CAD build for the part. Positions are in the model's coordinates, mm. Face numbers are marked on the shaded views. A direction names the side the tool comes from. Give positions to 0.01 mm unless a question says otherwise; leave off trailing zeros. Write each loop counter-clockwise with the first axis right and the second up, starting at its lowest first coordinate (ties: lowest second). Pieces come first, ordered by that corner, then holes. Notation, with made-up numbers: (-37, -1) -> (6, -1) arc R18 cw to (6, 26) -> close; hole circle Ø5 at (46, -11). An arc over 180 degrees is marked (long way). Answer as a JSON object with one key per item and string values.
```python
from build123d import *

# Parameters (mm, degrees)
F0_W     = 25
F0_H     = 38
F1_DEPTH = 5
F3_DEPTH = 5
F5_DEPTH = 15.5
F7_DEPTH = 25
F8_R     = 1.9
F9_DEPTH = 1


# Not quite as in the source:
# - a feature names something its author has since deleted; it is built from what else it names


with BuildPart() as f1:
    # F0 (on Top) → F1 (new body)
    with BuildSketch(Plane.XY):
        with Locations((-5.6626851261, 7.8445598302)):
            Rectangle(F0_W, F0_H)
    extrude(amount=F1_DEPTH)

    # F2 (on face) → F3 (cut)
    with BuildSketch(Plane.XY.offset(5)):
        with BuildLine():
            Line((-13.6626851261, 15.8445598302), (-12.5876851261, 15.8445598302))
            ThreePointArc((-12.5876851261, 15.8445598302), (-14.4228249158, 16.60469962), (-13.6626851261, 14.7695598302))
            Line((-13.6626851261, 14.7695598302), (-13.6626851261, 15.8445598302))
        make_face()
        with BuildLine():
            ThreePointArc((-13.6626851261, 14.7695598302), (-12.9025453363, 15.0844200404), (-12.5876851261, 15.8445598302))
            Line((-12.5876851261, 15.8445598302), (-13.6626851261, 15.8445598302))
            Line((-13.6626851261, 15.8445598302), (-13.6626851261, 14.7695598302))
        make_face()
        with BuildLine():
            Line((2.3373148739, 15.8445598302), (1.2623148739, 15.8445598302))
            ThreePointArc((1.2623148739, 15.8445598302), (1.5771750842, 15.0844200404), (2.3373148739, 14.7695598302))
            Line((2.3373148739, 14.7695598302), (2.3373148739, 15.8445598302))
        make_face()
        with BuildLine():
            ThreePointArc((3.4123148739, 15.8445598302), (2.3373148739, 16.9195598302), (1.2623148739, 15.8445598302))
            Line((1.2623148739, 15.8445598302), (2.3373148739, 15.8445598302))
            Line((2.3373148739, 15.8445598302), (2.3373148739, 14.7695598302))
            ThreePointArc((2.3373148739, 14.7695598302), (3.0974546637, 15.0844200404), (3.4123148739, 15.8445598302))
        make_face()
        with BuildLine():
            Line((-13.6626851261, -0.1554401698), (-13.6626851261, 0.9195598302))
            ThreePointArc((-13.6626851261, 0.9195598302), (-14.4228249158, -0.9155799596), (-12.5876851261, -0.1554401698))
            Line((-12.5876851261, -0.1554401698), (-13.6626851261, -0.1554401698))
        make_face()
        with BuildLine():
            ThreePointArc((-12.5876851261, -0.1554401698), (-12.9025453363, 0.60469962), (-13.6626851261, 0.9195598302))
            Line((-13.6626851261, 0.9195598302), (-13.6626851261, -0.1554401698))
            Line((-13.6626851261, -0.1554401698), (-12.5876851261, -0.1554401698))
        make_face()
        with BuildLine():
            Line((2.3373148739, -0.1554401698), (2.3373148739, 0.9195598302))
            ThreePointArc((2.3373148739, 0.9195598302), (1.5771750842, 0.60469962), (1.2623148739, -0.1554401698))
            Line((1.2623148739, -0.1554401698), (2.3373148739, -0.1554401698))
        make_face()
        with BuildLine():
            ThreePointArc((3.4123148739, -0.1554401698), (3.0974546637, 0.60469962), (2.3373148739, 0.9195598302))
            Line((2.3373148739, 0.9195598302), (2.3373148739, -0.1554401698))
            Line((2.3373148739, -0.1554401698), (1.2623148739, -0.1554401698))
            ThreePointArc((1.2623148739, -0.1554401698), (2.3373148739, -1.2304401698), (3.4123148739, -0.1554401698))
        make_face()
    extrude(amount=-F3_DEPTH, mode=Mode.SUBTRACT)

    # F4 (on face) → F5 (join)
    with BuildSketch(Plane.XY.offset(5)):
        Polygon((-15.2126851261, 13.8445598302), (-15.2126851261, 1.8445598302), (-14.2126851261, 1.8445598302), (-13.2126851261, 1.8445598302), (-13.2126851261, 13.8445598302), (-14.2126851261, 13.8445598302), align=None)
        Polygon((4.0873148739, 13.8445598302), (3.0873148739, 13.8445598302), (2.0873148739, 13.8445598302), (2.0873148739, 1.8445598302), (4.0873148739, 1.8445598302), align=None)
    extrude(amount=F5_DEPTH)

    # F6 (on face) → F7 (cut)
    with BuildSketch(Plane.YZ.offset(4.0873148739)):
        with BuildLine():
            Line((7.8445598302, 11.45), (7.8445598302, 14.55))
            ThreePointArc((7.8445598302, 14.55), (6.2945598302, 13), (7.8445598302, 11.45))
        make_face()
        with BuildLine():
            ThreePointArc((7.8445598302, 11.45), (8.9405753411, 11.9039844892), (9.3945598302, 13))
            ThreePointArc((9.3945598302, 13), (8.9405753411, 14.0960155108), (7.8445598302, 14.55))
            Line((7.8445598302, 14.55), (7.8445598302, 11.45))
        make_face()
    extrude(amount=-F7_DEPTH, mode=Mode.SUBTRACT)

    # F8 (on face) → F9 (cut)
    with BuildSketch(Plane.XY.offset(5)):
        with Locations((-13.6626851261, 15.8445598302)):
            Circle(F8_R)
        with Locations((2.3373148739, 15.8445598302)):
            Circle(F8_R)
        with Locations((2.3373148739, -0.1554401698)):
            Circle(F8_R)
        with Locations((-13.6626851261, -0.1554401698)):
            Circle(F8_R)
    extrude(amount=-F9_DEPTH, mode=Mode.SUBTRACT)


solid = f1.part
```
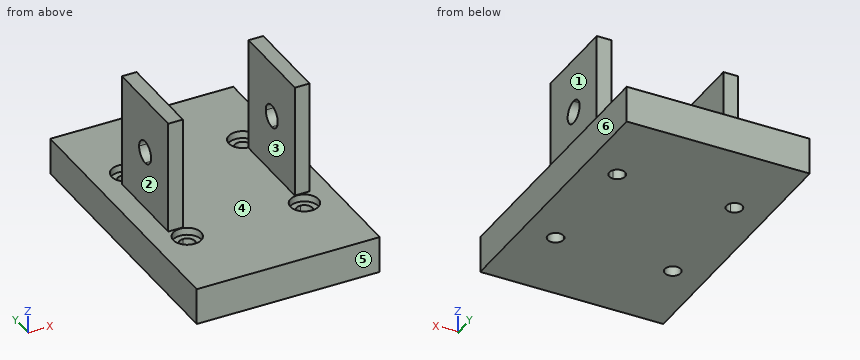
1) Slice it at B-B (z = 2.75). List the corners of the cut face in (x, y) (3 decimals).
Model answer:
{"outline": "(-18.163, -11.155) -> (6.837, -11.155) -> (6.837, 26.845) -> (-18.163, 26.845) -> close; hole circle Ø2.15 at (-13.663, -0.155); hole circle Ø2.15 at (-13.663, 15.845); hole circle Ø2.15 at (2.337, -0.155); hole circle Ø2.15 at (2.337, 15.845)"}
2) Wall check: probe 1 along X at (y, z) = (4, 13.75); probe 2 along Z at (x, y) = (2.5, 24.5); probe 3 along Y at (x, z) = (-13.5, 5.5). Give the ranges that are in metal, low to high.
Model answer:
{"probe 1": "x = -15.21 to -13.21, 2.09 to 4.09", "probe 2": "z = 0 to 5", "probe 3": "y = 1.84 to 13.84"}
3) Slice it at C-C (y = 5.5). List the corners of the cut face in (x, z).
Model answer:
{"outline": "(-18.16, 0) -> (6.84, 0) -> (6.84, 5) -> (4.09, 5) -> (4.09, 20.5) -> (2.09, 20.5) -> (2.09, 5) -> (-13.21, 5) -> (-13.21, 20.5) -> (-15.21, 20.5) -> (-15.21, 5) -> (-18.16, 5) -> close"}
4) Slice it at A-A (z = 7.25). List the corners of the cut face in (x, y).
Model answer:
{"outline": "(-15.21, 1.84) -> (-13.21, 1.84) -> (-13.21, 13.84) -> (-15.21, 13.84) -> close; (2.09, 1.84) -> (4.09, 1.84) -> (4.09, 13.84) -> (2.09, 13.84) -> close"}
5) 3-axis set-ups, long thin cutter, end or side, ignore diameter. For the marked faces 1, 2 and 3: which of +Z, -Z, +X, -X, +Y, -Y reach the whole face in a straight line?
Model answer:
{"face 1": "+Z, +X, +Y, -Y", "face 2": "+Z, -X, +Y, -Y", "face 3": "+Z, +Y, -Y"}
6) Pin check, flat tips, straight feed: pin 1 (8 mm diameter, centred on y = 4.5, z = 17.5, fed in from -X); pin 2 (1.1 mm diameter, centred on x = 3, y = 16, fed in from +Z); pin 3 (6 mm diameter, centred on x = -13.66, y = 15.84, fed in from -Z); pin 4 (0.6 mm diameter, centred on x = 2.5, z = 10, fed in from -Y). Stop position of each tip, or through.
Model answer:
{"pin 1": "stops at x = -15.21", "pin 2": "stops at z = 4", "pin 3": "stops at z = 0", "pin 4": "stops at y = 1.84"}
7) Mould opens along X. For the marked faces 4, 5 and 6 say: released by +X, released by -X, zero draft, split by the parting line, or undercut.
Model answer:
{"face 4": "undercut", "face 5": "zero draft", "face 6": "released by +X"}
8) Slice it at D-D (x = -3.75). List the corners of the cut face in (y, z).
Model answer:
{"outline": "(-11.16, 0) -> (26.84, 0) -> (26.84, 5) -> (-11.16, 5) -> close"}
